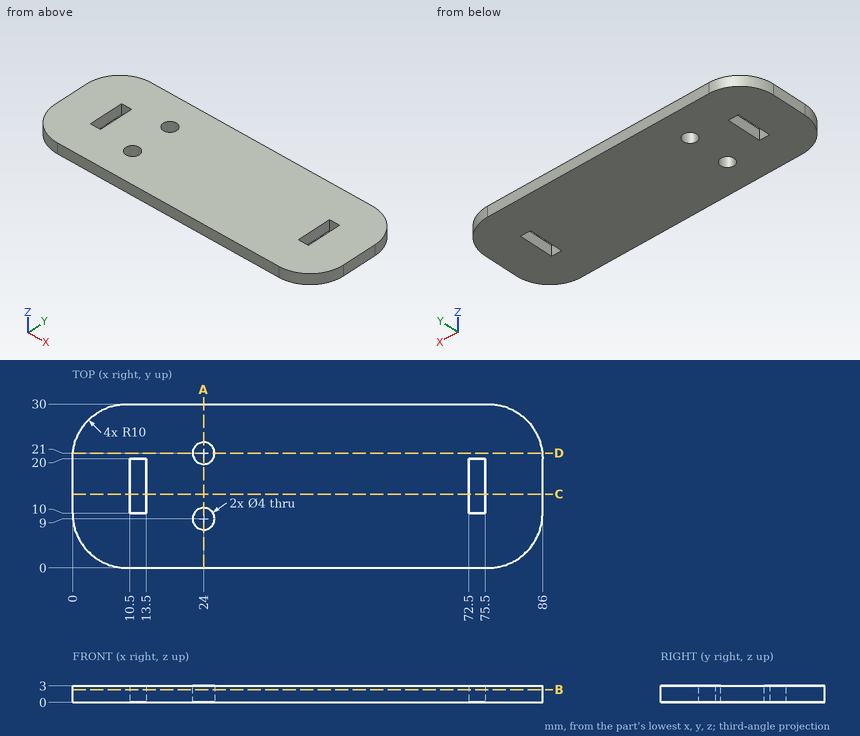
The figure shows three views and two pictorial views of one solid part (mm, origin at its lowest corner). Answer the questions. Give positions to 0.01 mm unless a question says otherwise; leave off trailing zeros. Loops run counter-clockwise (first coordinate to the right, second up) from the corner with the lowest first, then second, coordinate; pieces in that order, holes last. Notation, with made-up numbers: (4, 62) - (21, 62) arc R27 cw to (21, 96) - close; hole circle Ø10 at (-24, 11.5). An arc over 180 degrees is marked (long way). Use one line per item in the form item = value.
1. Find the intervals of material crossed by line 1 along Y through (x, z) = (24, 0.8); line 2 along X through (y, z) = (12, 1.5); line 3 along Y through (x, z) = (12, 0.3), in increasing order. Write a range as [from, to].
Calculated:
line_1 = [0, 7], [11, 19], [23, 30]
line_2 = [0, 10.5], [13.5, 72.5], [75.5, 86]
line_3 = [0, 10], [20, 30]
2. Section A-A on x = 24 is taken. Give the vertices of the cut face in (y, z).
Calculated:
outline = (0, 0) - (7, 0) - (7, 3) - (0, 3) - close; (11, 0) - (19, 0) - (19, 3) - (11, 3) - close; (23, 0) - (30, 0) - (30, 3) - (23, 3) - close
3. Section B-B on z = 2.35 is taken. Give the vertices of the cut face in (x, y), then the cut area to 3 significant figures.
Calculated:
outline = (0, 10) arc R10 ccw to (10, 0) - (76, 0) arc R10 ccw to (86, 10) - (86, 20) arc R10 ccw to (76, 30) - (10, 30) arc R10 ccw to (0, 20) - close; hole (10.5, 10) - (13.5, 10) - (13.5, 20) - (10.5, 20) - close; hole circle Ø4 at (24, 9); hole circle Ø4 at (24, 21); hole (72.5, 10) - (75.5, 10) - (75.5, 20) - (72.5, 20) - close
area = 2,410 mm^2
4. Section C-C on y = 13.5 is taken. Give the vertices of the cut face in (x, z), then the cut area to 3 significant figures.
Calculated:
outline = (0, 0) - (10.5, 0) - (10.5, 3) - (0, 3) - close; (13.5, 0) - (72.5, 0) - (72.5, 3) - (13.5, 3) - close; (75.5, 0) - (86, 0) - (86, 3) - (75.5, 3) - close
area = 240 mm^2
5. Section D-D on y = 21 is taken. Give the vertices of the cut face in (x, z), then the cut area to 3 significant figures.
Calculated:
outline = (0.05, 0) - (22, 0) - (22, 3) - (0.05, 3) - close; (26, 0) - (85.95, 0) - (85.95, 3) - (26, 3) - close
area = 246 mm^2
